Input: part model. Units: mm. Frame: model coordinates. Give positions to 0.01 mm unless a question says otherwise; leave off trailing zeros. Order: outer loops, then holes, each group sorted by start corner. A loop starts at its lowest first (then second) coordinate and runs counter-clockwise, first axis right, second up.
```python
from build123d import *

# Parameters (mm, degrees)
BOSS_EXTRUDE1_DEPTH = 5


with BuildPart() as part:
    # Sketch2 → Boss-Extrude1 (new body)
    with BuildSketch(Plane(origin=(0, 0, 0), x_dir=(1, 0, 0), z_dir=(0, 1, 0))):
        with BuildLine():
            Line((3.577708764, -7.155417528), (31.577708764, 6.844582472))
            ThreePointArc((31.577708764, 6.844582472), (32.561861408, 7.42813417), (33.452703386, 8.1461102))
            Line((33.452703386, 8.1461102), (38.402075473, 12.756285462))
            ThreePointArc((38.402075473, 12.756285462), (40.451835644, 14.048382243), (42.832396974, 14.5))
            Line((42.832396974, 14.5), (192.832396974, 14.5))
            ThreePointArc((192.832396974, 14.5), (197.428591052, 12.596194078), (199.332396974, 8))
            Line((199.332396974, 8), (199.332396974, -258))
            ThreePointArc((199.332396974, -258), (207.332396974, -266), (215.332396974, -258))
            Line((215.332396974, -258), (215.332396974, 8))
            ThreePointArc((215.332396974, 8), (217.236202896, 12.596194078), (221.832396974, 14.5))
            Line((221.832396974, 14.5), (477.167603026, 14.5))
            ThreePointArc((477.167603026, 14.5), (479.548164356, 14.048382243), (481.597924527, 12.756285462))
            Line((481.597924527, 12.756285462), (486.547296614, 8.1461102))
            ThreePointArc((486.547296614, 8.1461102), (499.44416276, 11.070078362), (492, 22))
            Line((492, 22), (28, 22))
            ThreePointArc((28, 22), (26.161976636, 21.785991916), (24.422291236, 21.155417528))
            Line((24.422291236, 21.155417528), (-3.577708764, 7.155417528))
            ThreePointArc((-3.577708764, 7.155417528), (-7.155417528, -3.577708764), (3.577708764, -7.155417528))
        make_face()
        with BuildLine():
            Line((2.906888371, -5.813776741), (30.906888371, 8.186223259))
            ThreePointArc((30.906888371, 8.186223259), (31.706512394, 8.660359013), (32.430321501, 9.243714538))
            Line((32.430321501, 9.243714538), (37.379693588, 13.8538898))
            ThreePointArc((37.379693588, 13.8538898), (39.902475337, 15.44416276), (42.832396974, 16))
            Line((42.832396974, 16), (192.832396974, 16))
            ThreePointArc((192.832396974, 16), (198.489251224, 13.656854249), (200.832396974, 8))
            Line((200.832396974, 8), (200.832396974, -258))
            ThreePointArc((200.832396974, -258), (207.332396974, -264.5), (213.832396974, -258))
            Line((213.832396974, -258), (213.832396974, 8))
            ThreePointArc((213.832396974, 8), (216.175542725, 13.656854249), (221.832396974, 16))
            Line((221.832396974, 16), (477.167603026, 16))
            ThreePointArc((477.167603026, 16), (480.097524663, 15.44416276), (482.620306412, 13.8538898))
            Line((482.620306412, 13.8538898), (487.569678499, 9.243714538))
            ThreePointArc((487.569678499, 9.243714538), (498.048382243, 11.61943867), (492, 20.5))
            Line((492, 20.5), (28, 20.5))
            ThreePointArc((28, 20.5), (26.506606016, 20.326118432), (25.093111629, 19.813776741))
            Line((25.093111629, 19.813776741), (-2.906888371, 5.813776741))
            ThreePointArc((-2.906888371, 5.813776741), (-5.813776741, -2.906888371), (2.906888371, -5.813776741))
        make_face(mode=Mode.SUBTRACT)
    extrude(amount=BOSS_EXTRUDE1_DEPTH)


solid = part.part
```
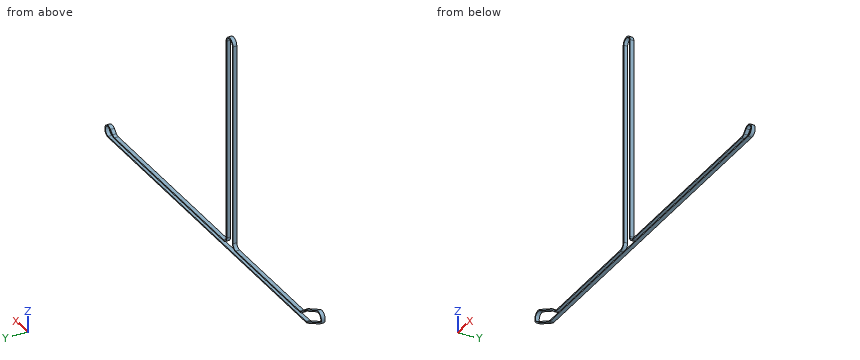
1) Cut plane A-A (x = 141.5). Return the cut outline in (y, z).
2) First-contact query: P1, Ø3, axis at y = 2.5, z = 220.5, coming from the +X side; P2, Ø2.5, axis at y = 3, z = 84.5, coming from the -X side; P3, Ø3, axis at x = 449, y = 4, coming from the +Z side; P4, Ø17, axis at x = 492, z = -14, coming from the +Y side. Flat tips, straight axial feed; report the tip coordinate or a pass-through.
3) Cut plane C-C (z = 0). Return the cut outline in (x, y).
4) Cut plane B-B (z = 89). Return the cut outline in (x, y).
5) Line query: probe 1 along X at (y, z) = (0.6, 164); probe 2 along Z at (x, y) = (239, 4.4); probe 3 along X at (y, z) = (3.85, -14). Output: solid intervals per line, ascending.
Geometry says:
1. outline: (0, -22) - (5, -22) - (5, -20.5) - (0, -20.5) - close; (0, -16) - (5, -16) - (5, -14.5) - (0, -14.5) - close
2. P1: stops at x = 215.33
2. P2: stops at x = 199.33
2. P3: stops at z = -14.5
2. P4: stops at y = 5
3. outline: (-8, 0) - (-6.5, 0) - (-6.5, 5) - (-8, 5) - close; (14.53, 0) - (17.89, 0) - (17.89, 5) - (14.53, 5) - close; (199.33, 0) - (200.83, 0) - (200.83, 5) - (199.33, 5) - close; (213.83, 0) - (215.33, 0) - (215.33, 5) - (213.83, 5) - close
4. outline: (199.33, 0) - (200.83, 0) - (200.83, 5) - (199.33, 5) - close; (213.83, 0) - (215.33, 0) - (215.33, 5) - (213.83, 5) - close
5. probe 1: x = 199.33 to 200.83, 213.83 to 215.33
5. probe 2: z = -22 to -20.5, -16 to -14.5
5. probe 3: x = 10.11 to 13.47, 37.54 to 40.33, 195.33 to 198.12, 216.54 to 219.33, 479.67 to 482.46, 498.5 to 500
